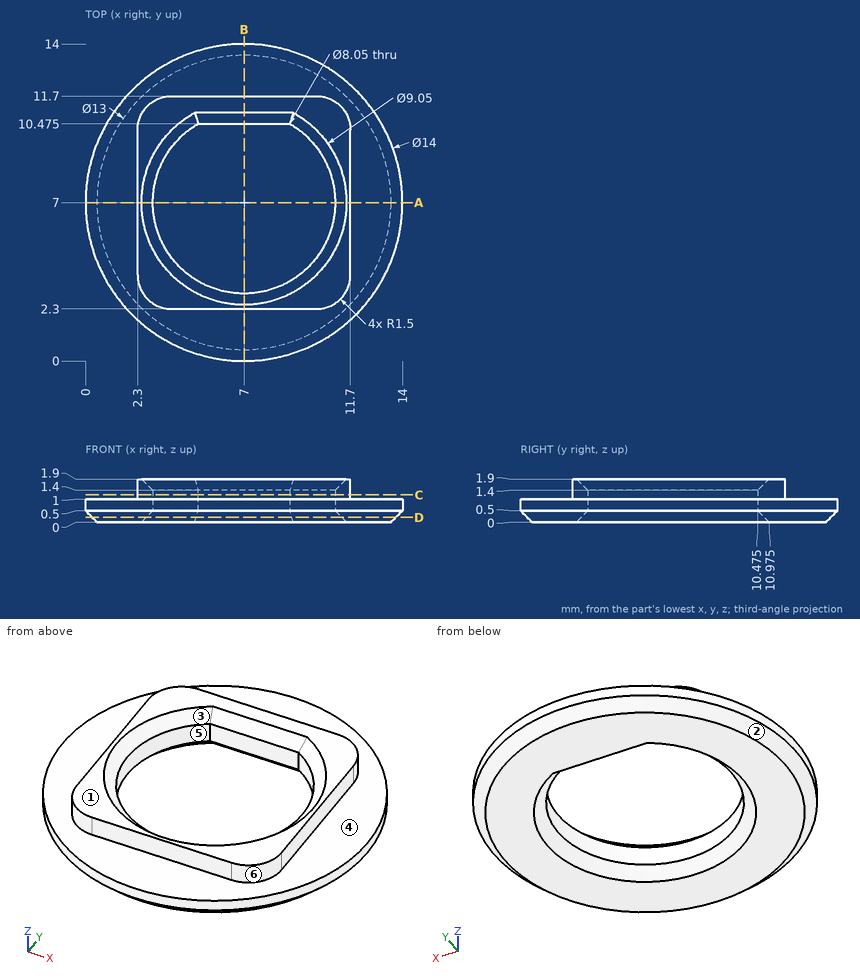
Print and shaded views of the part. All mm, measured from the part's lowest x, y and z. A direction names the side the tool comes from. Coordinates: 2 decimals unless noted, no trailing zeros. Write each loop counter-clockwise with the first axis right and the second up, starting at its lowest first coordinate (ties: lowest second). Pieces come first, ordered by that corner, then holes. Notation, with made-up numbers: (79, -38.5) -> (93, -38.5) arc R35 cw to (93, -3.5) -> close; hole circle Ø11 at (-19.5, 23.5). An arc over 180 degrees is marked (long way). Use CSV: the item, a comma, the result in double quotes. Start each with the question number.
Q1. 3-axis set-ups, long thin cutter, end or side, ignore diameter. For the marked faces 4, 5 and 6: which of +Z, -Z, +X, -X, +Y, -Y reach the whole face in a straight line?
Q2. Cut at C-C, the plane z = 1.2. List the corners of the cut face in (x, y) (3 decimals), then the cut area to 3 significant figures.
Q3. Cut at B-B, the plane x = 7. List the corners of the cut face in (y, z) (3 decimals), then the cut area to 3 significant figures.
Q4. Cut at A-A, the plane y = 7. List the corners of the cut face in (x, z) (3 decimals).
Q5. Cut at D-D, the plane z = 0.2. List the corners of the cut face in (x, y) (3 decimals).
Q6. Pull direction Y, two halves, no side cores. Call the marked faces 1, 2 and 3: released by +Y, released by -Y, zero draft, split by the parting line, or undercut.
Q7. Drill centre lines: probe 1 along Y at (x, z) = (7, 1.15) (3 decimals); probe 2 along Z at (x, y) = (6.25, 2); probe 3 along X at (y, z) = (4, 1.7). Where is each one in solid material? Low to high.
Q8. Flat gauge pins, fed straight in: pin 1 Ø1 at (x, z) = (5.5, 1) entering from +Y; pin 2 Ø1 at (x, y) = (6, 9) entering from -Z; pin 3 Ø5 at (x, y) = (10.5, 4.5) entering from -Z. Where does each tip first touch, or does it go through?
Checked values:
1,face 4,"+Z"
1,face 5,"+Z, -Z"
1,face 6,"+Z, +X, -Y"
2,outline,"(2.3, 3.8) arc R1.5 ccw to (3.8, 2.3) -> (10.2, 2.3) arc R1.5 ccw to (11.7, 3.8) -> (11.7, 10.2) arc R1.5 ccw to (10.2, 11.7) -> (3.8, 11.7) arc R1.5 ccw to (2.3, 10.2) -> close; hole (4.969, 10.475) arc R4.025 ccw (long way) to (9.031, 10.475) -> close"
2,area,"37.0 mm²"
3,outline,"(0, 0.5) -> (0.5, 0) -> (2.475, 0) -> (2.975, 0.5) -> (2.975, 1.4) -> (2.475, 1.9) -> (2.3, 1.9) -> (2.3, 1) -> (0, 1) -> close; (10.475, 0.5) -> (10.975, 0) -> (13.5, 0) -> (14, 0.5) -> (14, 1) -> (11.7, 1) -> (11.7, 1.9) -> (10.975, 1.9) -> (10.475, 1.4) -> close"
3,area,"7.46 mm²"
4,outline,"(0, 0.5) -> (0.5, 0) -> (2.475, 0) -> (2.975, 0.5) -> (2.975, 1.4) -> (2.475, 1.9) -> (2.3, 1.9) -> (2.3, 1) -> (0, 1) -> close; (11.025, 0.5) -> (11.525, 0) -> (13.5, 0) -> (14, 0.5) -> (14, 1) -> (11.7, 1) -> (11.7, 1.9) -> (11.525, 1.9) -> (11.025, 1.4) -> close"
5,outline,"circle Ø13.4 at (7, 7); hole (4.889, 10.775) arc R4.325 ccw (long way) to (9.111, 10.775) -> close"
6,face 1,"zero draft"
6,face 2,"split by the parting line"
6,face 3,"undercut"
7,probe 1,"y = 2.3 to 2.975, 10.475 to 11.7"
7,probe 2,"z = 0 to 1"
7,probe 3,"x = 2.3 to 3.88, 10.12 to 11.7"
8,pin 1,"stops at y = 13.93"
8,pin 2,"passes through"
8,pin 3,"stops at z = 0"
